from build123d import *

# Parameters (mm, degrees)
BOSS_EXTRUDE1_DEPTH     = 36
SKETCH2_R               = 2.625
CUT_EXTRUDE1_DEPTH      = 86.658085492
CUT_EXTRUDE2_DEPTH      = 94.206160811
CUT_EXTRUDE2_DEPTH_BACK = 94.206160811
SKETCH3_R               = 1.7


with BuildPart() as part:
    # Sketch1 → Boss-Extrude1 (new body)
    with BuildSketch(Plane.XY):
        Polygon((-42.618160568, 0.233338203), (-42.618160568, -9.766661797), (13.381839432, -9.766661797), (13.381839432, 65.233338203), (-16.742848795, 65.233338203), (-16.742848795, 0.233338203), align=None)
    extrude(amount=BOSS_EXTRUDE1_DEPTH)

    # Sketch2 → Cut-Extrude1 (cut, through all)
    with BuildSketch(Plane(origin=(0, 0.233338203, 0), x_dir=(1, 0, 0), z_dir=(0, 1, 0))):
        with Locations(Location((-29.680504682, -18, 0), (0, 0, 270))):
            Circle(SKETCH2_R)
    extrude(amount=-CUT_EXTRUDE1_DEPTH, mode=Mode.SUBTRACT)

    # Sketch3 → Cut-Extrude2 (cut, two sides: drawn at the far end of the back side and taken through both)
    with BuildSketch(Plane(origin=(13.381839432, 0, 0), x_dir=(0, 0, -1), z_dir=(1, 0, 0)).offset(-CUT_EXTRUDE2_DEPTH_BACK)):
        with Locations((-24.687630005, 20.233338203)):
            Circle(SKETCH3_R)
        with Locations((-10.520088066, 20.233338203)):
            Circle(SKETCH3_R)
        with Locations((-24.687630005, 42.461110081)):
            Circle(SKETCH3_R)
        with Locations((-10.520088066, 42.461110081)):
            Circle(SKETCH3_R)
    extrude(amount=CUT_EXTRUDE2_DEPTH + CUT_EXTRUDE2_DEPTH_BACK, mode=Mode.SUBTRACT)


solid = part.part
Part model, mm, in its own coordinate system. A direction names the side the tool comes from. Coordinates: 2 decimals unless noted, no trailing zeros. Loops run counter-clockwise (first coordinate to the right, second up) from the corner with the lowest first, then second, coordinate; pieces in that order, holes last. Notation, with made-up numbers: (-25.5, 21) -> (11.5, 21) arc R6 ccw to (11.5, 31) -> close; hole circle Ø10 at (-24.5, -3). An arc over 180 degrees is marked (long way). Use a Markdown table: item, result. Add a question column.
Item 1: Band-saw the part on D-D on z = 25. Write the cut outline in (x, y), plus the area to 3 significant figures.
Item 2: Band-saw the part on C-C on z = 7. Write the cut outline in (x, y).
Item 3: Which spindle directions (+Z, -Z, +X, -X, +Y, -Y) get a long thin tool onto all of the face, cutting with end or side? Do faces 1 (the flat face through (-26.6, 0.233, 17.7)), 2 (the flat face through (-42.618, -5, 18)). Say none if no direction does.
Item 4: Band-saw the part on A-A on z = 18. Write the cut outline in (x, y).
Item 5: Flat gauge pins, fed straight in: P1, Ø3, axis at y = 42.46, z = 24.69, coming from the -X side; P2, Ø6, axis at x = -29.68, z = 18, coming from the +Y side; P3, Ø11, axis at y = 27.5, z = 19, coming from the -X side. Where does each tip first touch, or does it go through?
Item 6: Pull direction X, two halves, no side cores. Call faces 3 (the flat face through (-16.743, 33, 18)), 4 (the cylindrical face through (-32.243, -4.697, 17.431)), 5 (the cylindrical face through (-1.89, 41.81, 8.95)): +X half, -X half, draft (parallel to the pull), parting line (faces both ways), or undercut.
Item 7: Probe probe 1 along Y at (x, z) = (-7, 10); probe 2 along X at (y, z) = (53, 27); probe 3 along X at (y, z) = (-2.5, 18). List the from-to ranges inside material, lowest first.
Item 8: Band-saw the part on B-B on x = -28.5. Write the cut outline in (y, z), plus the area to 3 significant figures.
Geometry says:
| question | item | result |
|---|---|---|
| 1 | outline | (-42.62, -9.77) -> (13.38, -9.77) -> (13.38, 18.56) -> (-16.74, 18.56) -> (-16.74, 0.23) -> (-42.62, 0.23) -> close; (-16.74, 21.9) -> (13.38, 21.9) -> (13.38, 40.79) -> (-16.74, 40.79) -> close; (-16.74, 44.13) -> (13.38, 44.13) -> (13.38, 65.23) -> (-16.74, 65.23) -> close |
| 1 | area | 2,320 mm² |
| 2 | outline | (-42.62, -9.77) -> (13.38, -9.77) -> (13.38, 65.23) -> (-16.74, 65.23) -> (-16.74, 0.23) -> (-42.62, 0.23) -> close |
| 3 | face 1 | +Z, -Z, -X, +Y |
| 3 | face 2 | +Z, -Z, -X, +Y, -Y |
| 4 | outline | (-42.62, -9.77) -> (-32.31, -9.77) -> (-32.31, 0.23) -> (-42.62, 0.23) -> close; (-27.06, -9.77) -> (13.38, -9.77) -> (13.38, 65.23) -> (-16.74, 65.23) -> (-16.74, 0.23) -> (-27.06, 0.23) -> close |
| 5 | P1 | through |
| 5 | P2 | y = 0.23 |
| 5 | P3 | x = -16.74 |
| 6 | face 3 | -X half |
| 6 | face 4 | undercut |
| 6 | face 5 | draft |
| 7 | probe 1 | -9.77 to 18.61, 21.85 to 40.84, 44.08 to 65.23 |
| 7 | probe 2 | -16.74 to 13.38 |
| 7 | probe 3 | -42.62 to -32.31, -27.06 to 13.38 |
| 8 | outline | (-9.77, 0) -> (0.23, 0) -> (0.23, 15.66) -> (-9.77, 15.66) -> close; (-9.77, 20.34) -> (0.23, 20.34) -> (0.23, 36) -> (-9.77, 36) -> close |
| 8 | area | 313 mm² |
